Build history of the part. All positions in model axes, mm. Face numbers are marked on the shaded views. Coordinates: 2 decimals unless noted, no trailing zeros. Write each loop counter-clockwise with the first axis right and the second up, starting at its lowest first coordinate (ties: lowest second). Pieces come first, ordered by that corner, then holes.
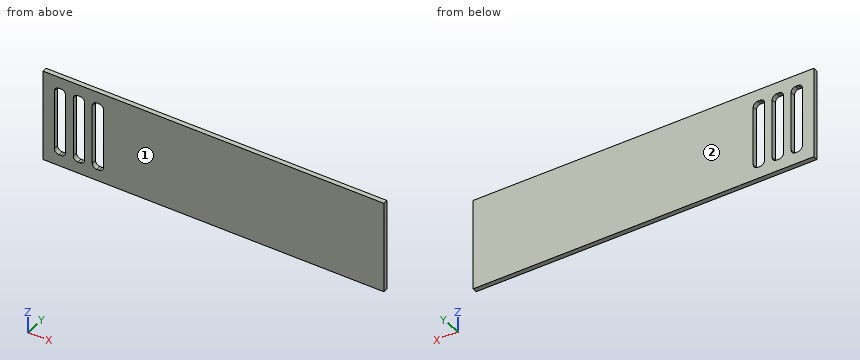
from build123d import *

# Parameters (mm, degrees)
SKETCH1_W               = 450
SKETCH1_H               = 120
BOSS_EXTRUDE1_DEPTH     = 6.35
SKETCH2_W               = 15
SKETCH2_H               = 90
CUT_EXTRUDE1_DEPTH      = 1
CUT_EXTRUDE1_DEPTH_BACK = 7.35
FILLET1_R               = 6


with BuildPart() as part:
    # Sketch1 → Boss-Extrude1 (new body)
    with BuildSketch(Plane(origin=(0, 0, 0), x_dir=(1, 0, 0), z_dir=(0, 1, 0))):
        with Locations((225, 60)):
            Rectangle(SKETCH1_W, SKETCH1_H)
    extrude(amount=BOSS_EXTRUDE1_DEPTH)

    # Sketch2 → Cut-Extrude1 (cut, two sides)
    with BuildSketch(Plane(origin=(0, 6.35, 0), x_dir=(1, 0, 0), z_dir=(0, 1, 0))) as cut_extrude1_sk:
        with Locations((22.5, 60)):
            Rectangle(SKETCH2_W, SKETCH2_H)
        with Locations((47.5, 60)):
            Rectangle(SKETCH2_W, SKETCH2_H)
        with Locations((72.5, 60)):
            Rectangle(SKETCH2_W, SKETCH2_H)
    extrude(amount=CUT_EXTRUDE1_DEPTH, mode=Mode.SUBTRACT)
    extrude(cut_extrude1_sk.sketch, amount=-CUT_EXTRUDE1_DEPTH_BACK, mode=Mode.SUBTRACT)

    # Fillet1
    fillet1_edges = [part.edges().sort_by_distance(p)[0] for p in [
        (15, 3.175, -105),
        (30, 3.175, -105),
        (30, 3.175, -15),
        (15, 3.175, -15),
        (65, 3.175, -105),
        (80, 3.175, -105),
        (80, 3.175, -15),
        (65, 3.175, -15),
        (40, 3.175, -15),
        (40, 3.175, -105),
        (55, 3.175, -105),
        (55, 3.175, -15),
    ]]
    fillet(fillet1_edges, radius=FILLET1_R)


solid = part.part
(1) Slice it at A-A, the plane z = -66.5. List the corners of the cut face in (x, y), and give its area (3 significant figures).
(2) Slice it at B-B, the plane y = 2. List the corners of the cut face in (x, z).
(3) Probe L1, parallel to X at y = 0.5, z = -79; L2, parallel to X at y = 2.5, z = -102; L3, parallel to Z at x = 44, y = 4.75. List the from-to ranges inside material, lowest first.
(4) Two-plate mould, pull along Y, no slides. Class the marked faces 1 and 2: pulls with the +Y half, pulls with the -Y half, needs draft (parallel to the pull), parting line crosses it, or undercut.
Results:
1. outline: (0, 0) - (15, 0) - (15, 6.35) - (0, 6.35) - close; (30, 0) - (40, 0) - (40, 6.35) - (30, 6.35) - close; (55, 0) - (65, 0) - (65, 6.35) - (55, 6.35) - close; (80, 0) - (450, 0) - (450, 6.35) - (80, 6.35) - close
1. area: 2,570 mm2
2. outline: (0, -120) - (450, -120) - (450, 0) - (0, 0) - close; hole (15, -99) arc R6 ccw to (21, -105) - (24, -105) arc R6 ccw to (30, -99) - (30, -21) arc R6 ccw to (24, -15) - (21, -15) arc R6 ccw to (15, -21) - close; hole (40, -99) arc R6 ccw to (46, -105) - (49, -105) arc R6 ccw to (55, -99) - (55, -21) arc R6 ccw to (49, -15) - (46, -15) arc R6 ccw to (40, -21) - close; hole (65, -99) arc R6 ccw to (71, -105) - (74, -105) arc R6 ccw to (80, -99) - (80, -21) arc R6 ccw to (74, -15) - (71, -15) arc R6 ccw to (65, -21) - close
3. L1: x = 0 to 15, 30 to 40, 55 to 65, 80 to 450
3. L2: x = 0 to 15.8, 29.2 to 40.8, 54.2 to 65.8, 79.2 to 450
3. L3: z = -120 to -104.66, -15.34 to 0
4. face 1: pulls with the -Y half
4. face 2: pulls with the +Y half
